For this review, take the finished solid that the model builds, in its own axes (mm). Round coordinates to 2 decimals unless told otherwise and drop trailing zeros. Order: outer loops, then holes, each group sorted by start corner. A loop starts at its lowest first (then second) coordinate and runs counter-clockwise, first axis right, second up. Notation, with made-up numbers: M 21,31.5 L 65,31.5 A15 cw 65,50.5 Z; hole C 61,-15 d3. An arc over 180 degrees is marked long. Put each result on its own line as item: value.
from build123d import *

# Parameters (mm, degrees)
F0_R      = 76.2
F1_DEPTH  = 25.4
F2_R      = 5.08
F1_FACE_R = 71.12
F3_DEPTH  = 6.35


with BuildPart() as f1:
    # F0 (on Front) → F1 (new body)
    with BuildSketch(Plane.XZ):
        Circle(F0_R)
    extrude(amount=F1_DEPTH)

    # F2
    f2_edges = [f1.edges().sort_by_distance(p)[0] for p in [
        (-76.2, -25.4, 0),
    ]]
    fillet(f2_edges, radius=F2_R)

    # F1_face (on face) → F3 (cut)
    with BuildSketch(Plane.XZ.offset(25.4)):
        Circle(F1_FACE_R)
    extrude(amount=-F3_DEPTH, mode=Mode.SUBTRACT)


solid = f1.part
(1) Add section C-C on y = -6. Give the boundary of the cut face in (x, z).
A:
outline: C 0,0 d152.4
(2) Add section A-A on x = 0. Give the boundary of the cut face in (y, z), then the cut area to 3 significant figures.
A:
outline: M -25.4,-71.12 A5.08 ccw -20.32,-76.2 L 0,-76.2 L 0,76.2 L -20.32,76.2 A5.08 ccw -25.4,71.12 L -19.05,71.12 L -19.05,-71.12 Z
area: 2,960 mm2
(3) Add section B-B on z = 0. Give the boundary of the cut face in (x, y), then the cut area to 3 significant figures.
A:
outline: M -76.2,-20.32 A5.08 ccw -71.12,-25.4 L -71.12,-19.05 L 71.12,-19.05 L 71.12,-25.4 A5.08 ccw 76.2,-20.32 L 76.2,0 L -76.2,0 Z
area: 2,960 mm2
(4) To check wall thickness, follow L1, parallel to Y at x = 20, z = -6; L2, parallel to Z at x = 3, y = -23; L3, parallel to Z at x = 0, y = -22. State the ranges of each line that lie inside material, in increasing order.
A:
L1: y = -19.05 to 0
L2: z = -75.38 to -71.06, 71.06 to 75.38
L3: z = -75.91 to -71.12, 71.12 to 75.91
(5) Insertion check: pin 1 Ø6 at (x, z) = (-34.5, -43.5) entering from -Y; pin 2 Ø2 at (x, y) = (-41, -13.5) entering from -Z; pin 3 Ø6 at (x, y) = (-24.5, -16) entering from +Z. Each pin has a flat end and moves straight along its axis. Give the tip position at first contact, or say it passes through.
A:
pin 1: stops at y = -19.05
pin 2: stops at z = -64.86
pin 3: stops at z = 73.1
(6) Draft analysis for pull direction X (two halves, no side actions). For faces 1 (the face through (-60.47, -10.018, -46.367)), 2 (the face through (-15.42, -22.27, -69.43)), 3 (the face through (-1, -19.05, 1)), 4 (the face through (-1, 0, 1)), state which applies: released by +X, released by -X, zero draft, split by the parting line, or undercut.
A:
face 1: split by the parting line
face 2: undercut
face 3: undercut
face 4: zero draft
